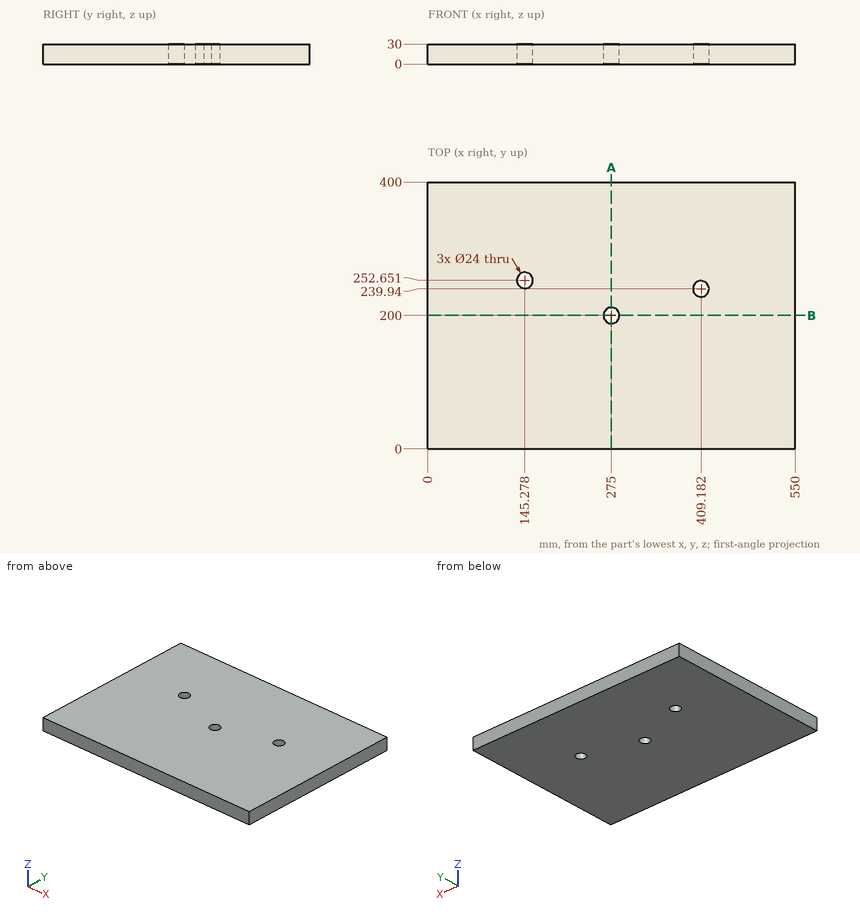
Design review of the part shown in the three views and the two pictorial views. Dimensions are in mm from the part's minimum x, y and z. Coordinates: 2 decimals unless noted, no trailing zeros. Order: outer loops, then holes, each group sorted by start corner. A loop starts at its lowest first (then second) coordinate and runs counter-clockwise, first axis right, second up. Notation, with made-up numbers: (81.5, 57.25) -> (130.5, 57.25) arc R13 cw to (130.5, 82.25) -> close; hole circle Ø11 at (69.25, -4). An arc over 180 degrees is marked (long way). Use one line per item in the form item = value. Start each with the question number.
(1) Add section A-A on x = 275. State the section outline as (y, z) points, plus the area to 3 significant figures.
(2) For probe 1 along Y at (x, z) = (275, 14); probe 2 along Y at (x, z) = (404, 28) (1 decimal), list the stretches that pass through material, from the lowest coordinate up.
(3) Add section B-B on y = 200. State the section outline as (x, z) points, plus the area to 3 significant figures.
Answer block:
q1.outline = (0, 0) -> (188, 0) -> (188, 30) -> (0, 30) -> close; (212, 0) -> (400, 0) -> (400, 30) -> (212, 30) -> close
q1.area = 11,300 mm²
q2.probe_1 = 0 to 188, 212 to 400
q2.probe_2 = 0 to 229.1, 250.8 to 400
q3.outline = (0, 0) -> (263, 0) -> (263, 30) -> (0, 30) -> close; (287, 0) -> (550, 0) -> (550, 30) -> (287, 30) -> close
q3.area = 15,800 mm²
